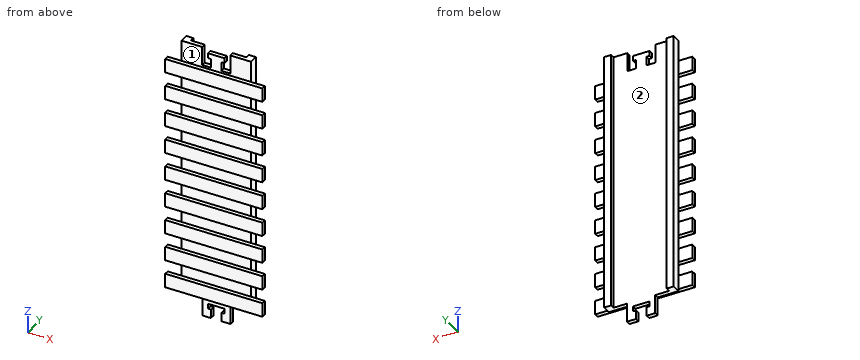
```python
from build123d import *

# Parameters (mm, degrees)
F1_DEPTH = 3.175
F2_W     = 50.8
F2_H     = 10.1607441902
F2_W_2   = 10.16
F2_H_2   = 10.16
F2_H_3   = 10.1088657975
F2_H_4   = 10.2023631334
F3_DEPTH = 3.175
F2_H_5   = 10.2422460914
F4_DEPTH = 3.175
F5_W     = 5.1035365641
F5_H     = 189.5493796663
F5_W_2   = 5.0522950478
F6_DEPTH = 3.175


with BuildPart() as f1:
    # F0 (on Front) → F1 (new body)
    with BuildSketch(Plane.XZ):
        with BuildLine():
            Line((25.5517161727, -116.6203990579), (15.2647161727, -116.6203990579))
            Line((15.2647161727, -116.6203990579), (15.2647161727, -130.2710193916))
            Line((15.2647161727, -130.2710193916), (21.4880950641, -130.2710193916))
            ThreePointArc((21.4880950641, -130.2710193916), (21.5113434052, -129.8451671692), (21.5808121, -129.4243766025))
            Line((21.5808121, -129.4243766025), (21.5808121, -123.7957928851))
            Line((21.5808121, -123.7957928851), (19.3710121, -123.7957928851))
            Line((19.3710121, -123.7957928851), (19.3710121, -120.0983975604))
            Line((19.3710121, -120.0983975604), (31.5819798807, -120.0983975604))
            Line((31.5819798807, -120.0983975604), (31.5819798807, -123.7957928851))
            Line((31.5819798807, -123.7957928851), (29.3721798807, -123.7957928851))
            Line((29.3721798807, -123.7957928851), (29.3721798807, -130.2710193916))
            Line((29.3721798807, -130.2710193916), (35.8426272869, -130.2710193916))
            Line((35.8426272869, -130.2710193916), (35.8426272869, -116.6203990579))
            Line((35.8426272869, -116.6203990579), (25.5517161727, -116.6203990579))
        make_face()
        Polygon((15.113, 72.9289806084), (0, 72.9289806084), (0, -116.6203990579), (15.2647161727, -116.6203990579), (25.5517161727, -116.6203990579), (35.8426272869, -116.6203990579), (50.8, -116.6203990579), (50.8, 72.9289806084), (35.6909111142, 72.9289806084), (35.6909111142, 59.2783602747), (29.220463708, 59.2783602747), (29.220463708, 65.7749548554), (31.430263708, 65.7749548554), (31.430263708, 69.4723501801), (19.3802, 69.4723501801), (19.3802, 65.7749548554), (21.59, 65.7749548554), (21.59, 59.2783602747), (15.113, 59.2783602747), align=None)
    extrude(amount=F1_DEPTH)

    # F2 (on face) → F3 (join)
    with BuildSketch(Plane.XZ.offset(3.175)):
        with Locations((25.4, 52.5756378829)):
            Rectangle(F2_W, F2_H)
        with Locations((55.88, 52.5756378829)):
            Rectangle(F2_W_2, F2_H)
        with Locations((-5.08, 52.5756378829)):
            Rectangle(F2_W_2, F2_H)
        with Locations((-5.08, 32.2552657878)):
            Rectangle(F2_W_2, F2_H_2)
        with Locations((25.4, 32.2552657878)):
            Rectangle(F2_W, F2_H_2)
        with Locations((55.88, 32.2552657878)):
            Rectangle(F2_W_2, F2_H_2)
        with Locations((55.88, 11.9352657878)):
            Rectangle(F2_W_2, F2_H_2)
        with Locations((25.4, 11.9352657878)):
            Rectangle(F2_W, F2_H_2)
        with Locations((-5.08, 11.9352657878)):
            Rectangle(F2_W_2, F2_H_2)
        with Locations((-5.08, -8.3847342122)):
            Rectangle(F2_W_2, F2_H_2)
        with Locations((25.4, -8.3847342122)):
            Rectangle(F2_W, F2_H_2)
        with Locations((55.88, -8.3847342122)):
            Rectangle(F2_W_2, F2_H_2)
        with Locations((55.88, -28.7047342122)):
            Rectangle(F2_W_2, F2_H_2)
        with Locations((25.4, -28.7047342122)):
            Rectangle(F2_W, F2_H_2)
        with Locations((-5.08, -28.7047342122)):
            Rectangle(F2_W_2, F2_H_2)
        with Locations((-5.08, -49.0247342122)):
            Rectangle(F2_W_2, F2_H_2)
        with Locations((25.4, -49.0247342122)):
            Rectangle(F2_W, F2_H_2)
        with Locations((55.88, -49.0247342122)):
            Rectangle(F2_W_2, F2_H_2)
        with Locations((55.88, -69.310028106)):
            Rectangle(F2_W_2, F2_H_3)
        with Locations((25.4, -69.310028106)):
            Rectangle(F2_W, F2_H_3)
        with Locations((-5.08, -69.310028106)):
            Rectangle(F2_W_2, F2_H_3)
        with Locations((-5.08, -89.587919414)):
            Rectangle(F2_W_2, F2_H_4)
        with Locations((25.4, -89.587919414)):
            Rectangle(F2_W, F2_H_4)
        with Locations((55.88, -89.587919414)):
            Rectangle(F2_W_2, F2_H_4)
    extrude(amount=F3_DEPTH)

    # F2 (on face) → F4 (join)
    with BuildSketch(Plane.XZ.offset(3.175)):
        with Locations((25.4, -110.0125946105)):
            Rectangle(F2_W, F2_H_5)
        with Locations((55.88, -110.0125946105)):
            Rectangle(F2_W_2, F2_H_5)
        with Locations((-5.08, -110.0125946105)):
            Rectangle(F2_W_2, F2_H_5)
    extrude(amount=F4_DEPTH)

    # F5 (on face) → F6 (join)
    with BuildSketch(Plane(origin=(0, 0, 0), x_dir=(-1, 0, 0), z_dir=(0, 1, 0))):
        with Locations((-48.2482317179, -21.8457092247)):
            Rectangle(F5_W, F5_H)
        with Locations((-2.5261475239, -21.8457092247)):
            Rectangle(F5_W_2, F5_H)
    extrude(amount=F6_DEPTH)


solid = f1.part
```
The model under review builds one solid part; all positions refer to its coordinate system, in mm. Face numbers are marked on the shaded views. A direction names the side the tool comes from. Coordinates: 2 decimals unless noted, no trailing zeros. Write each loop counter-clockwise with the first axis right and the second up, starting at its lowest first coordinate (ties: lowest second). Pieces come first, ordered by that corner, then holes.
1) Clearance check with flat-ended pins moving along their axes: pin 1 Ø3.5 at (x, y) = (39.5, -5) entering from -Z; pin 2 Ø5 at (x, z) = (55.5, -89) entering from +Y (3 decimals); pin 3 Ø2.5 at (x, y) = (33, -5) entering from +Z; pin 4 Ø1.5 at (x, y) = (10.5, 1) entering from +Z. State where each tip first meets the part, or that it passes through.
2) We need section D-D on z = 20. State the section outline as (x, y) points (3 decimals), then the cut area to 3 significant figures.
3) We need section C-C on x = 56. Count the separate pieces of the cut face and the enclosed holes in it, then the cut area to 3 significant figures.
4) To check wall thickness, follow probe 1 along X at (y, z) = (1, -22); probe 2 along X at (y, z) = (-2.25, -55.5); probe 3 along Y at (x, z) = (8.5, -35) (3 decimals). State the ranges of each line that lie inside material, in increasing order.
5) We need section A-A on y = 1.5. State the section outline as (x, z) points.
6) We need section B-B on z = -27. State the section outline as (x, y) points (3 decimals).
7) Machinability: for the marked faces 1 and 2, which of the approach directions +Z, -Z, +X, -X, +Y, -Y give a long, thin tool a straight path to every point of the face, cutting with its end or side? Answer none if there is none.
Answer list:
1. pin 1: stops at z = -115.13
1. pin 2: stops at y = -3.175
1. pin 3: stops at z = 57.66
1. pin 4: passes through
2. outline: (0, -3.175) - (50.8, -3.175) - (50.8, 3.175) - (45.696, 3.175) - (45.696, 0) - (5.052, 0) - (5.052, 3.175) - (0, 3.175) - close
2. area: 194 mm2
3. separate pieces: 9
3. enclosed holes: 0
3. area: 291 mm2
4. probe 1: x = 0 to 5.05, 45.7 to 50.8
4. probe 2: x = 0 to 50.8
4. probe 3: y = -3.175 to 0
5. outline: (0, -116.62) - (5.05, -116.62) - (5.05, 72.93) - (0, 72.93) - close; (45.7, -116.62) - (50.8, -116.62) - (50.8, 72.93) - (45.7, 72.93) - close
6. outline: (-10.16, -6.35) - (60.96, -6.35) - (60.96, -3.175) - (50.8, -3.175) - (50.8, 3.175) - (45.696, 3.175) - (45.696, 0) - (5.052, 0) - (5.052, 3.175) - (0, 3.175) - (0, -3.175) - (-10.16, -3.175) - close
7. face 1: +Z, +X, -X, -Y
7. face 2: +Z, -Z, +Y
